Check sheet for the modelled part. Datum: model origin and axes. Units: mm. A direction names the side the tool comes from. Coordinates: 2 decimals unless noted, no trailing zeros. Loops run counter-clockwise (first coordinate to the right, second up) from the corner with the lowest first, then second, coordinate; pieces in that order, holes last.
```python
from build123d import *

# Parameters (mm, degrees)
F0_W     = 30
F0_H     = 45
F1_DEPTH = 25
F3_D     = 7.1374
F4_R     = 5
F5_DEPTH = 9.2
F6_DEPTH = 8.8


with BuildPart() as f1:
    # F0 (on Front) → F1 (new body)
    with BuildSketch(Plane.XZ):
        with Locations((15, 22.5)):
            Rectangle(F0_W, F0_H)
    extrude(amount=F1_DEPTH)

    # F3 (through all)
    with Locations(Plane.XZ.offset(25)):
        with Locations((15, 22.5)):
            Hole(F3_D / 2)

    # F4
    f4_edges = [f1.edges().sort_by_distance(p)[0] for p in [
        (30, -12.5, 45),
        (0, -12.5, 45),
    ]]
    fillet(f4_edges, radius=F4_R)

    # F5 (add): a face of the model
    f5_faces = [f1.faces().sort_by_distance(p)[0] for p in [
        (30, -12.5, 20),
    ]]
    extrude(f5_faces, amount=F5_DEPTH)

    # F6 (add): a face of the model
    f6_faces = [f1.faces().sort_by_distance(p)[0] for p in [
        (0, -12.5, 20),
    ]]
    extrude(f6_faces, amount=F6_DEPTH)


solid = f1.part
```
1) Scan lines: line 1 (Z direction, x = 15, y = -14); line 2 (Z direction, x = 31.5, y = -10); line 3 (X direction, y = -22.75, z = 23.5). Record each from-to range of solid material in increasing order.
Answer sheet:
line 1: z = 0 to 18.93, 26.07 to 45
line 2: z = 0 to 40
line 3: x = -8.8 to 11.57, 18.43 to 39.2
2) Depth check by flat-ended pin: pin 1 (4.5 mm diameter, centred on x = 35.5, y = -13, fed in from +Z). Enter the tip coordinate at first touch or a pass-through.
Answer sheet:
pin 1: stops at z = 40
3) Section check C-C on y = -3.25. Enter the section's corners in (x, z), plus the area to 3 significant figures.
Answer sheet:
outline: (-8.8, 0) - (39.2, 0) - (39.2, 40) - (30, 40) arc R5 ccw to (25, 45) - (5, 45) arc R5 ccw to (0, 40) - (-8.8, 40) - close; hole circle Ø7.14 at (15, 22.5)
area: 2,020 mm2
4) Section check A-A on x = 15. Enter the section's corners in (y, z).
Answer sheet:
outline: (-25, 0) - (0, 0) - (0, 18.93) - (-25, 18.93) - close; (-25, 26.07) - (0, 26.07) - (0, 45) - (-25, 45) - close
5) Section check B-B on z = 22.5. Enter the section's corners in (x, y), plus the area to 3 significant figures.
Answer sheet:
outline: (-8.8, -25) - (11.43, -25) - (11.43, 0) - (-8.8, 0) - close; (18.57, -25) - (39.2, -25) - (39.2, 0) - (18.57, 0) - close
area: 1,020 mm2
6) Section check D-D on x = 33. Enter the section's corners in (y, z), plus the area to 3 significant figures.
Answer sheet:
outline: (-25, 0) - (0, 0) - (0, 40) - (-25, 40) - close
area: 1,000 mm2
7) Set-up check for faces 4 (the flat face through (35, -12, 40)), 5 (the flat face through (16, 0, 17)), 6 (the flat face through (-4, -12, 40)): record each of +Z, -Z, +X, -X, +Y, -Y from which the full face is reachable in a straight line by a thin tool's end or side.
Answer sheet:
face 4: +Z, +X, +Y, -Y
face 5: +Z, -Z, +X, -X, +Y
face 6: +Z, -X, +Y, -Y
8) Mould release check, pull along Z, two halves, no side actions. Record for faces 1 (the flat face through (16, -25, 17)), 2 (the cylindrical face through (15.774, -12.325, 19.016)), 3 (the flat face through (15, -12, 45)): +Z half, -Z half, draft (parallel to the pull), parting line (faces both ways), or undercut.
Answer sheet:
face 1: draft
face 2: undercut
face 3: +Z half
